Verification items for the finished model (mm, model axes). A direction names the side the tool comes from. Round coordinates to 2 decimals unless told otherwise and drop trailing zeros. Loops run counter-clockwise (first coordinate to the right, second up) from the corner with the lowest first, then second, coordinate; pieces in that order, holes last. Notation, with made-up numbers: (15, -38.75) -> (69, -38.75) arc R26 ccw to (69, -5.75) -> close; hole circle Ø11 at (5, 36). An arc over 180 degrees is marked (long way). Write item = value, one per line.
Autodesk Inventor part; units mm, degrees
ref_plane "Work Plane1" through (0, 5.4991, 0) normal (0, 1, 0) x (-1, 0, 0)
ref_plane "YZ Plane" through (0, 0, 0) normal (1, 0, 0) x (0, 1, 0)
ref_plane "XY Plane" through (0, 0, 0) normal (0, 0, 1) x (1, 0, 0)
sketch "Sketch1" plane through (0, 0, 0) normal (0, 0, 1) x (1, 0, 0)
  circle A0 centre (0, 0) radius 5.4991
  dimension "d0" = 10.9982
extrude "Extrusion1" add sketch "Sketch1" against normal blind 6.604
chamfer "Chamfer1" distance 0.254 angle 45 2 edges at (-5.4991, 0, 0) (-5.4991, 0, -6.604)
sketch "Sketch2" plane through (0, 0, 0) normal (0, 0, 1) x (1, 0, 0)
  circle A0 centre (0, 0) radius 5.2451
hole "Hole1" at (0, 0, 0) direction (0, 0, -1) diameter 4.191 end through all
ref_plane "Work Plane1" through (0, 5.4991, 0) normal (0, 1, 0) x (-1, 0, 0)
sketch "Sketch3" plane through (0, 5.4991, 0) normal (0, 1, 0) x (-1, 0, 0)
  line L0 (-5.2451, 0) -> (5.2451, 0)
  line L1 (5.4991, -0.254) -> (5.4991, -6.35)
  point P0 (0, 0)
  point P1 (0, -3.302)
hole "Hole2" at (0, 5.4991, -3.302) direction (0, -1, 0) diameter 3.302 end up to surface
chamfer "Chamfer2" distance 0.254 angle 45 2 edges at (0, 2.0955, 0) (0, 2.0955, -6.604)
properties part number "Shaft Collar"
(1) Material ranges on probe 1 along Y at (x, z) = (0, -1.5); probe 2 along Z at (x, y) = (0, 2.5); probe 3 along X at (y, z) = (4.75, -4), recorded low to high. Write a range as from..to.
Filled sheet:
probe_1 = -5.5..-2.1, 2.1..5.5
probe_2 = -6.6..-4.95, -1.65..0
probe_3 = -2.77..-1.5, 1.5..2.77
(2) Set-up check for faces 4 (the face through (1.1, -2.3, -6.604)), 5 (the face through (-0.07, 3.83, -4.95)): record each of +Z, -Z, +X, -X, +Y, -Y from which the full face is reachable in a straight line by a thin tool's end or side.
Filled sheet:
face_4 = -Z, +X, -X, +Y, -Y
face_5 = +Y
(3) Go/stop test with a flat-tipped pin: pin 1 Ø1 at (y, z) = (1, -5) entering from -X. Record where the tip stops, or that it passes through.
Filled sheet:
pin_1 = -5.48
(4) Draft check along Y on faces 1 (the face through (-1.19, -5.37, -3.26)), 2 (the face through (1.1, -2.3, 0)), 3 (the face through (0.803, -1.936, -3.345)). Enter one of: released by +Y, released by -Y, zero draft, split by the parting line, or undercut.
Filled sheet:
face_1 = split by the parting line
face_2 = zero draft
face_3 = undercut
(5) Sectioned sample at D-D, the plane z = -4.75. Record the cut outline in (x, y), and give its area (3 significant figures).
Filled sheet:
outline = (-0.79, 1.94) -> (-0.79, 5.44) arc R5.5 ccw (long way) to (0.79, 5.44) -> (0.79, 1.94) arc R2.1 cw (long way) to start
area = 75.8 mm2
(6) Sectioned sample at B-B, the plane y = 0. Record the cut outline in (x, z).
Filled sheet:
outline = (-5.5, -6.35) -> (-5.25, -6.6) -> (-2.35, -6.6) -> (-2.1, -6.35) -> (-2.1, -0.25) -> (-2.35, 0) -> (-5.25, 0) -> (-5.5, -0.25) -> close; (2.1, -6.35) -> (2.35, -6.6) -> (5.25, -6.6) -> (5.5, -6.35) -> (5.5, -0.25) -> (5.25, 0) -> (2.35, 0) -> (2.1, -0.25) -> close
(7) Sectioned sample at C-C, the plane z = -1. Record the cut outline in (x, y), and give its area (3 significant figures).
Filled sheet:
outline = circle Ø11 at (0, 0); hole circle Ø4.19 at (0, 0)
area = 81.2 mm2
(8) Sectioned sample at A-A, the plane x = 0. Record the cut outline in (y, z).
Filled sheet:
outline = (-5.5, -6.35) -> (-5.25, -6.6) -> (-2.35, -6.6) -> (-2.1, -6.35) -> (-2.1, -0.25) -> (-2.35, 0) -> (-5.25, 0) -> (-5.5, -0.25) -> close; (2.1, -6.35) -> (2.35, -6.6) -> (5.25, -6.6) -> (5.5, -6.35) -> (5.5, -4.95) -> (2.1, -4.95) -> close; (2.1, -1.65) -> (5.5, -1.65) -> (5.5, -0.25) -> (5.25, 0) -> (2.35, 0) -> (2.1, -0.25) -> close
